from build123d import *

# Parameters (mm, degrees)
F0_W     = 508
F0_H     = 419.1
F1_DEPTH = 19.05
F2_W     = 508
F2_H     = 6.35
F3_DEPTH = 12.7
F4_R     = 6.35
F5_DEPTH = 19.051


# Not quite as in the source:
# - a pattern or mirror of a feature is missing from the dataset's text; its kind, count and spacing are read off the source's solid


with BuildPart() as f1:
    # F0 (on Top) → F1 (new body)
    with BuildSketch(Plane.XY):
        Rectangle(F0_W, F0_H)
    extrude(amount=F1_DEPTH)

    # F2 (on face) → F3 (cut)
    with BuildSketch(Plane.XZ.offset(209.55)):
        with Locations((0, 3.175)):
            Rectangle(F2_W, F2_H)
        with Locations((0, 15.875)):
            Rectangle(F2_W, F2_H)
    f3 = extrude(amount=-F3_DEPTH, mode=Mode.SUBTRACT)

    # F3_copies: F3 across plane
    add(f3.mirror(Plane.ZX), mode=Mode.SUBTRACT)

    # F4 (on face) → F5 (cut, through all)
    with BuildSketch(Plane.XY.offset(19.05)):
        Circle(F4_R)
    extrude(amount=-F5_DEPTH, mode=Mode.SUBTRACT)


solid = f1.part
The listing builds one solid part. Answer for the finished solid, in the listing's coordinates (mm). A direction names the side the tool comes from. Give positions to 0.01 mm unless a question says otherwise; leave off trailing zeros. Write each loop counter-clockwise with the first axis right and the second up, starting at its lowest first coordinate (ties: lowest second). Pieces come first, ordered by that corner, then holes. Notation, with made-up numbers: (49.5, 54) -> (79.5, 54) arc R14 ccw to (79.5, 75) -> close; hole circle Ø7 at (47.25, 68). An arc over 180 degrees is marked (long way). One line per question, with ' | ' between items. Start each with the question number.
1. Section B-B (x = 0) is taken. Determine the outline of the cut face in (y, z).
2. For a pull along Y with two mould halves and no side action, classify faces 1 (the flat face through (-254, -3, 9)), 2 (the cylindrical face through (-1.38, -6.2, 9.66)) as pulls with the +Y half, pulls with the -Y half, needs draft (parallel to the pull), parting line crosses it, or undercut.
3. Section C-C (x = 209) is taken. Determine the outline of the cut face in (y, z).
4. Find the intervals of material crossed by probe 1 along Y at (x, z) = (0, 15); probe 2 along Y at (x, z) = (0, 10.25); probe 3 along Y at (x, z) = (-100.5, 2.5), in increasing order.
5. Section A-A (y = 0) is taken. Determine the outline of the cut face in (x, z).
6. Given pin 1 Ø14 at (x, y) = (6.5, 206) entering from +Z; pin 2 Ø5 at (x, z) = (-94.5, 15.5) entering from +Y; pin 3 Ø2 at (x, z) = (-129, 4.5) entering from -Y, each flat-ended and moving along its own axis, determine where each tip first touches the part or whether it passes through.
7. For faces 3 (the flat face through (-4, 203, 6.35)), 4 (the flat face through (-4, -203, 12.7)), 5 (the flat face through (-4, 203, 12.7)), 6 (the flat face through (-4, -203, 6.35)), determine the directions among +Z, -Z, +X, -X, +Y, -Y from which every point of the face is accessible in a straight line to the end or side of a thin tool.
Response values:
1) outline: (-209.55, 6.35) -> (-196.85, 6.35) -> (-196.85, 0) -> (-6.35, 0) -> (-6.35, 19.05) -> (-196.85, 19.05) -> (-196.85, 12.7) -> (-209.55, 12.7) -> close; (6.35, 0) -> (196.85, 0) -> (196.85, 6.35) -> (209.55, 6.35) -> (209.55, 12.7) -> (196.85, 12.7) -> (196.85, 19.05) -> (6.35, 19.05) -> close
2) face 1: needs draft | face 2: undercut
3) outline: (-209.55, 6.35) -> (-196.85, 6.35) -> (-196.85, 0) -> (196.85, 0) -> (196.85, 6.35) -> (209.55, 6.35) -> (209.55, 12.7) -> (196.85, 12.7) -> (196.85, 19.05) -> (-196.85, 19.05) -> (-196.85, 12.7) -> (-209.55, 12.7) -> close
4) probe 1: -196.85 to -6.35, 6.35 to 196.85 | probe 2: -209.55 to -6.35, 6.35 to 209.55 | probe 3: -196.85 to 196.85
5) outline: (-254, 0) -> (-6.35, 0) -> (-6.35, 19.05) -> (-254, 19.05) -> close; (6.35, 0) -> (254, 0) -> (254, 19.05) -> (6.35, 19.05) -> close
6) pin 1: z = 12.7 | pin 2: y = 196.85 | pin 3: y = -196.85
7) face 3: -Z, +X, -X, +Y | face 4: +Z, +X, -X, -Y | face 5: +Z, +X, -X, +Y | face 6: -Z, +X, -X, -Y
